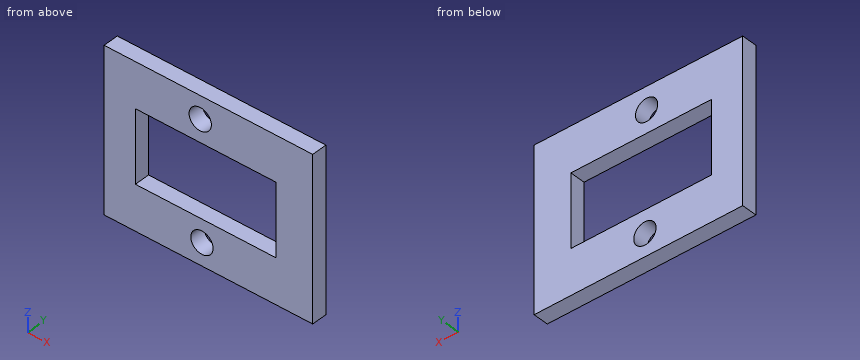
```python
from build123d import *

# Parameters (mm, degrees)
SKETCH2_W           = 34.12443
SKETCH2_H           = 26.478152769
SKETCH2_R           = 1.825
SKETCH2_W_2         = 23
SKETCH2_H_2         = 11.79979
BOSS_EXTRUDE1_DEPTH = 1.25


with BuildPart() as part:
    # Sketch2 → Boss-Extrude1 (new, symmetric)
    with BuildSketch(Plane(origin=(0, 0, 0), x_dir=(1, 0, 0), z_dir=(0, 1, 0))):
        with Locations((0.360723362, 0.777502601)):
            Rectangle(SKETCH2_W, SKETCH2_H)
        with Locations(Location((-0.702610465, 10.366481865, 0), (0, 0, 270))):
            Circle(SKETCH2_R, mode=Mode.SUBTRACT)
        with Locations(Location((-0.97805, -8.773518135, 0), (0, 0, 270))):
            Circle(SKETCH2_R, mode=Mode.SUBTRACT)
        with Locations((-0.088760873, 0.7809876)):
            Rectangle(SKETCH2_W_2, SKETCH2_H_2, mode=Mode.SUBTRACT)
    extrude(amount=BOSS_EXTRUDE1_DEPTH, both=True)


solid = part.part
```
Work out the finished part from the listing and answer in its coordinate system (mm). Give positions to 0.01 mm unless a question says otherwise; leave off trailing zeros. Write each loop counter-clockwise with the first axis right and the second up, starting at its lowest first coordinate (ties: lowest second). Pieces come first, ordered by that corner, then holes. Notation, with made-up numbers: (-18.75, -4.5) -> (-13.75, -4.5) arc R24 ccw to (-13.75, 10.5) -> close; hole circle Ø1 at (-30, 54.25). An arc over 180 degrees is marked (long way). Write item = value, one per line.
Q1. Section C-C on y = 0.15 is taken. State how many separate pieces and enclosed holes the cut face has, and give its area (3 significant figures).
Computed values:
separate_pieces = 1
enclosed_holes = 3
area = 611 mm^2
Q2. Consider line 1 along Z through (x, y) = (-5.5, -1.1); line 2 along Z through (x, y) = (-1, 0.8); line 3 along X through (y, z) = (0.1, 1.75). Determine where each line is inside the solid, lowest interval first.
Computed values:
line_1 = -14.02 to -6.68, 5.12 to 12.46
line_2 = -14.02 to -12.17, -8.57 to -6.68, 5.12 to 6.95, 10.6 to 12.46
line_3 = -16.7 to -11.59, 11.41 to 17.42
Q3. Section B-B on x = -8.5 is taken. Determine the outline of the cut face in (y, z).
Computed values:
outline = (-1.25, -14.02) -> (1.25, -14.02) -> (1.25, -6.68) -> (-1.25, -6.68) -> close; (-1.25, 5.12) -> (1.25, 5.12) -> (1.25, 12.46) -> (-1.25, 12.46) -> close
Q4. Section A-A on z = -1.5 is taken. Determine the outline of the cut face in (x, y), and give its area (3 significant figures).
Computed values:
outline = (-16.7, -1.25) -> (-11.59, -1.25) -> (-11.59, 1.25) -> (-16.7, 1.25) -> close; (11.41, -1.25) -> (17.42, -1.25) -> (17.42, 1.25) -> (11.41, 1.25) -> close
area = 27.8 mm^2
Q5. Flat-ended cylindrical pins translate along their axes: pin 1 Ø3.5 at (x, z) = (-0.98, 8.77) entering from -Y; pin 2 Ø5 at (x, z) = (-9.5, -4) entering from -Y. Find the tip coordinate at first contact, or state that the pin passes through.
Computed values:
pin_1 = through
pin_2 = -1.25
